Input: part model. Units: mm. Frame: model coordinates. Coordinates: 2 decimals unless noted, no trailing zeros.
Item 1: Contact query for flat-ended pins moving along their axis: P1, Ø5, axis at y = -12, z = 28, coming from the -X side; P2, Ø3, axis at y = -12, z = -28, coming from the -X side. Output: stop coordinate, or through.
Item 2: Ray query, line 1 along Z through (x, y) = (-0.6, 12.5); line 2 along Z through (x, y) = (0.65, 12); line 3 along Y through (x, z) = (0.7, -28). Return the intervals inside material, ascending.
Item 3: Section A-A on x = 0.6. Give the number of separate pieces and of enclosed holes in the cut face, and give its area (3 significant figures).
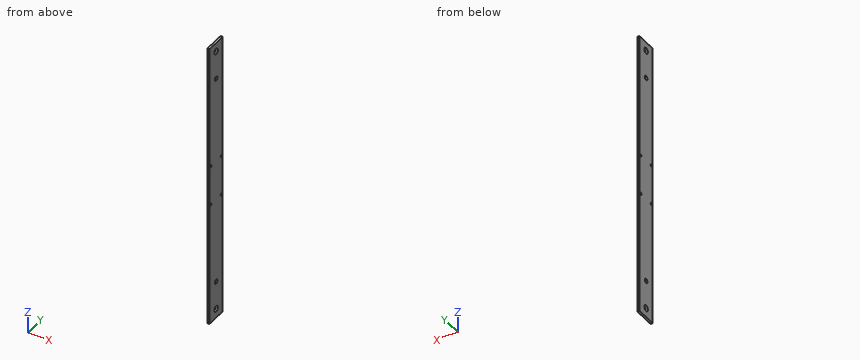
Autodesk Inventor part; units mm, degrees
ref_plane "YZ Plane" through (0, 0, 0) normal (1, 0, 0) x (0, 1, 0)
ref_plane "XZ Plane" through (0, 0, 0) normal (0, 1, 0) x (-1, 0, 0)
ref_plane "XY Plane" through (0, 0, 0) normal (0, 0, 1) x (1, 0, 0)
sketch "Sketch2" plane through (-1.5, 0, 0) normal (-1, 0, 0) x (0, 0, 1)
  circle A0 centre (177.25, 0.2229) radius 2.55
  circle A1 centre (157.25, 0.2229) radius 2.55
  point P0 (0, 0)
sketch "Sketch1" plane through (0, 0, 0) normal (1, 0, 0) x (0, 1, 0)
  line L0 (15, 200) -> (-15, 200)
  line L1 (-15, 200) -> (-15, -200)
  line L2 (-15, -200) -> (15, -200)
  line L3 (15, -200) -> (15, 200)
  line L4 (15, 200) -> (-15, -200) construction
  line L5 (-15, 200) -> (15, -200) construction
  point P0 (0, 0)
  point P1 (0, 0)
  dimension "d0" = 400
  dimension "d1" = 30
extrude "Plate1" add sketch "Sketch1" along normal mid plane 3
sketch "Sketch3" plane through (-1.5, 0, 0) normal (-1, 0, 0) x (0, 0, 1)
  circle A0 centre (187.6, 0) radius 4
  circle A1 centre (147.9, 0) radius 3
  circle A2 centre (-147.4, 0) radius 3
  circle A3 centre (-187.1, 0) radius 4
  line L0 (200, 15) -> (200, -15)
  line L1 (-200, -15) -> (-200, 15)
  line L2 (200, -15) -> (-200, -15)
  point P0 (0, 0)
  dimension "d7" = 12.4
  dimension "d8" = 8
  dimension "d9" = 39.7
  dimension "d10" = 6
  dimension "d22" = 8
  dimension "d23" = 6
  dimension "d24" = 12.9
  dimension "d26" = 15
  dimension "d27" = 39.7
extrude "Cut2" cut sketch "Sketch3" against normal blind 3
sketch "Sketch4" plane through (1.5, 0, 0) normal (1, 0, 0) x (0, 0, -1)
  line L0 (-200, 15) -> (200, 15)
  point P0 (0, 0)
  point P1 (-28, 12)
  point P2 (-28, -12)
  point P3 (28, 12)
  point P4 (28, -12)
  dimension "d11" = 56
  dimension "d12" = 24
  dimension "d13" = 3
  dimension "d14" = 28
hole "Hole1" at (1.5, 12, 28) at (1.5, -12, 28) at (1.5, 12, -28) at (1.5, -12, -28) direction (-1, 0, 0) diameter 3.242 depth 11.8 tip angle 118
equation "\"d27\" = d9"
equation "\"d5\" = Thickness"
equation "\"d2\" = Thickness"
equation "\"BendRadius\" = Thickness"
equation "\"BendReliefWidth\" = Thickness"
equation "\"BendReliefDepth\" = 0.5 * Thickness"
equation "\"CornerReliefSize\" = 4 * Thickness"
equation "\"MinimumRemnant\" = 2 * Thickness"
equation "\"TransitionRadius\" = BendRadius"
equation "\"JacobiRadiusSize\" = BendRadius"
equation "\"GapSize\" = Thickness"
properties part number "HCMUTE-CDT23-OP_DVCAM" material "PMMA Plastic"
Results found:
1. P1: stops at x = -1.5
1. P2: passes through
2. line 1: z = -200 to -29.54, -26.46 to 26.46, 29.54 to 200
2. line 2: z = -200 to -29.62, -26.38 to 26.38, 29.62 to 200
2. line 3: y = -15 to -13.62, -10.38 to 10.38, 13.62 to 15
3. separate pieces: 1
3. enclosed holes: 8
3. area: 11,800 mm2
